```python
from build123d import *

# Parameters (mm, degrees)
F1_DEPTH    = 5
F2_T1_DEPTH = 22.6347624906


# Not quite as in the source:
# - a fillet or chamfer that OpenCascade refuses, or shapes differently, is made with other operations: its cross-section is extruded or revolved along the edge and cut away or added


with BuildPart() as f1:
    # F0 (on Top) → F1 (new body)
    with BuildSketch(Plane.XY):
        with BuildLine():
            ThreePointArc((5.9922465209, -7.8176391342), (-9.8492732487, 0.1196514659), (6.1803914025, 7.6697628458))
            Line((6.1803914025, 7.6697628458), (7.9372539332, 9.85))
            ThreePointArc((7.9372539332, 9.85), (-11.9294802904, 4.2083250825), (0, -12.65))
            ThreePointArc((0, -12.65), (8.8388347648, -16.3111652352), (12.5, -25.15))
            ThreePointArc((12.5, -25.15), (2.7054951742, -37.353700089), (-11.328847338, -30.4327282718))
            Line((-11.328847338, -30.4327282718), (-16.1166251075, -20.1653057112))
            Line((-16.1166251075, -20.1653057112), (-18.6542869112, -21.3486368441))
            Line((-18.6542869112, -21.3486368441), (-13.8665091417, -31.6160594046))
            ThreePointArc((-13.8665091417, -31.6160594046), (7.9338387883, -38.2322093731), (12.1431348989, -15.8422465209))
            Line((12.1431348989, -15.8422465209), (7.5500579161, -9.85))
            Line((7.5500579161, -9.85), (5.9922465209, -7.8176391342))
        make_face()
    extrude(amount=F1_DEPTH)

    # F2: fillet of radius 3.6213203436 on 1 edges, made by hand

    # F2_s2 → F2_t1 (cut)
    with BuildSketch(Plane.XY.offset(-8.8173812453)):
        with BuildLine():
            ThreePointArc((-14.6260705735, -23.3618102248), (-16.289199108, -21.6529383212), (-18.6542869112, -21.3486368441))
            Line((-18.6542869112, -21.3486368441), (-16.1166251075, -20.1653057112))
            Line((-16.1166251075, -20.1653057112), (-14.6260705735, -23.3618102248))
        make_face()
    extrude(amount=F2_T1_DEPTH, mode=Mode.SUBTRACT)


solid = f1.part
```
Can you work these out from the model? Positions are in its coordinate system, mm. A direction names the side the tool comes from. Round coordinates to 2 decimals unless told otherwise and drop trailing zeros. Order: outer loops, then holes, each group sorted by start corner. A loop starts at its lowest first (then second) coordinate and runs counter-clockwise, first axis right, second up. Notation, with made-up numbers: (89.25, 47.25) -> (100.25, 47.25) arc R34 ccw to (100.25, 81.25) -> close; hole circle Ø11 at (5.5, 12.25). An arc over 180 degrees is marked (long way). Return JSON: item names as keys, results as strings. Group by question number.
1. We'd pull the mould along X, two halves only. Please class faces 4 (the face through (7.624, -38.415, 2.465)), 5 (the face through (-9.85, -0.19, 2.46)), 6 (the face through (-16.259, -21.668, 2.465)), 7 (the face through (-2, -12, 0)): released by +X, released by -X, zero draft, split by the parting line, or undercut.
2. Which directions (+Z, -Z, +X, -X, +Y, -Y) give clear straight access to the entire face, cutting with the end or side of a thin tool? Please do faces 1 (the face through (7.047, 8.745, 2.465)), 2 (the face through (-12.954, -26.947, 2.465)), 3 (the face through (-2, -12, 5)).
3. I need wall thicknesses on line 1 (Y direction, x = -1, z = 3.1); line 2 (Y direction, x = 1, z = 2.35); line 3 (X direction, y = 0, z = 3.3). Which ranges of each line are inside material? Lowest first, please. Write a range as [from, to].
4. If we section it at A-A, the plane y = -36: Write out the boundary of the cut face in (x, z), then the cut area to 3 significant figures.
5. If we section it at D-D, the plane x = 11.5: Write out the boundary of the cut face in (y, z), then the cut area to 3 significant figures.
6. Will these pins go through, and if not, where does the flat tip stop? pin 1 (2 mm diameter, centred on x = 10.5, z = 2, fed in from +Y); pin 2 (1 mm diameter, centred on x = -5.5, z = 4.5, fed in from -Y).
7. If we section it at C-C, the plane z = 4.05: Write out the boundary of the cut face in (x, y).
8. If we section it at B-B, the plane x = 3: Write out the boundary of the cut face in (y, z), then the cut area to 3 significant figures.
Output values:
{
 "1": {"face 4": "split by the parting line", "face 5": "undercut", "face 6": "undercut", "face 7": "zero draft"},
 "2": {"face 1": "+Z, -Z, +X", "face 2": "+Z, -Z", "face 3": "+Z, +X, -X, +Y, -Y"},
 "3": {"line 1": "[-40.42, -37.61], [-12.61, -9.8], [9.8, 12.61]", "line 2": "[-40.42, -37.61], [-12.69, -9.8], [9.8, 12.61]", "line 3": "[-12.65, -9.85]"},
 "4": {"outline": "(-10.79, 0) -> (-6.21, 0) -> (-6.21, 5) -> (-10.79, 5) -> close; (6.21, 0) -> (10.79, 0) -> (10.79, 5) -> (6.21, 5) -> close", "area": "45.8 mm²"},
 "5": {"outline": "(-35.24, 0) -> (-30.05, 0) -> (-30.05, 5) -> (-35.24, 5) -> close; (-20.25, 0) -> (-15, 0) -> (-15, 5) -> (-20.25, 5) -> close", "area": "52.2 mm²"},
 "6": {"pin 1": "y = -12.39", "pin 2": "y = -39.61"},
 "7": {"outline": "(-18.65, -21.35) -> (-13.87, -31.62) arc R15.3 ccw (long way) to (12.14, -15.84) -> (5.99, -7.82) arc R9.85 cw (long way) to (6.18, 7.67) -> (7.94, 9.85) arc R12.65 ccw (long way) to (0, -12.65) arc R12.5 cw (long way) to (-11.33, -30.43) -> (-14.63, -23.36) arc R3.62 ccw to start"},
 "8": {"outline": "(-40.15, 0) -> (-37.28, 0) -> (-37.28, 5) -> (-40.15, 5) -> close; (-13.02, 0) -> (-9.38, 0) -> (-9.38, 5) -> (-13.02, 5) -> close; (9.38, 0) -> (12.29, 0) -> (12.29, 5) -> (9.38, 5) -> close", "area": "47.0 mm²"}
}
